Design review of the part built by this model. Coordinates are the model's own, in mm. Face numbers are marked on the shaded views. Coordinates: 2 decimals unless noted, no trailing zeros. Write each loop counter-clockwise with the first axis right and the second up, starting at its lowest first coordinate (ties: lowest second). Pieces come first, ordered by that corner, then holes.
Q1. The part is to be moulded in two halves that separate along X. For the marked faces 1, 2 and 3, say which applies: +X half, -X half, draft (parallel to the pull), parting line (faces both ways), or undercut.
Q2. Clearance check with flat-ended pins moving along their axes: pin 1 Ø1.6 at (x, z) = (-43, 35) entering from +Y; pin 2 Ø1.5 at (x, y) = (-95, 1) entering from -Z; pin 3 Ø1 at (y, z) = (-0.5, 27) entering from +X; pin 4 Ø1.5 at (x, y) = (-46, -1.5) entering from -Z. State where each tip first meets the part, or that it passes through.
Q3. Add section D-D, the plane x = -70. Give the boundary of the cut face in (y, z), plus the area to 3 significant figures.
Q4. To check wall thickness, follow probe 1 along Z at (x, y) = (-43, 0.65); probe 2 along X at (y, z) = (0.85, 35); probe 3 along Z at (x, y) = (-89.5, -1.6). State the ranges of each line that lie inside material, in increasing order.
Q5. Add section B-B, the plane y = -0.3. Give the boundary of the cut face in (x, z), plus the area to 3 significant figures.
Q6. Add section C-C, the plane z = 7. Give the boundary of the cut face in (x, y), plus the area to 3 significant figures.
Q7. Add section A-A, the plane x = -103. Give the boundary of the cut face in (y, z).
from build123d import *

# Parameters (mm, degrees)
SKETCH_R     = 1
PAD_DEPTH    = 4
POCKET_DEPTH = 0.5


with BuildPart() as part:
    # Sketch → Pad (new body)
    with BuildSketch(Plane(origin=(-43, 2, 10), x_dir=(-1, 0, 0), z_dir=(0, -1, 0))):
        with BuildLine():
            ThreePointArc((1.369567, -6.241771), (-2.39195, -6.793979), (-3.992648, -10.242416))
            Line((-3.992648, -10.242416), (-3.999699, -25.049081))
            ThreePointArc((-3.999699, -25.049081), (0.10526, -28.998615), (3.996742, -24.838581))
            Line((3.996742, -24.838581), (6.436421, -15.831628))
            ThreePointArc((10.468861, -13.107373), (8.040921, -13.860073), (6.436421, -15.831628))
            ThreePointArc((10.468861, -13.107373), (37.233561, -5.679802), (61.911635, 7.068166))
            ThreePointArc((61.911635, 7.068166), (63.070989, 11.678996), (58.563715, 13.191721))
            ThreePointArc((1.369567, -6.241771), (31.05105, 0.283484), (58.563715, 13.191721))
        make_face()
        with Locations((0, -10)):
            Circle(SKETCH_R, mode=Mode.SUBTRACT)
        with Locations((60, 10)):
            Circle(SKETCH_R, mode=Mode.SUBTRACT)
        with Locations((0, -25)):
            Circle(SKETCH_R, mode=Mode.SUBTRACT)
    extrude(amount=PAD_DEPTH)

    # Sketch001 → Pocket (cut)
    with BuildSketch(Plane(origin=(-43, -2, 10), x_dir=(-1, 0, 0), z_dir=(0, -1, 0))):
        with BuildLine():
            ThreePointArc((-0.032814, -13.479149), (2.709829, -12.250672), (3.417072, -9.329876))
            ThreePointArc((4.97037, -6.903931), (3.291608, -7.539293), (3.417072, -9.329876))
            ThreePointArc((4.97037, -6.903931), (30.091825, -0.923478), (53.929252, 9.007808))
            ThreePointArc((56.670903, 5.328015), (57.272793, 8.637695), (53.929252, 9.007808))
            ThreePointArc((9.344748, -11.398275), (33.841325, -5.393473), (56.670903, 5.328015))
            ThreePointArc((9.344748, -11.398275), (6.419172, -12.709963), (4.685346, -15.40688))
            Line((4.685346, -15.40688), (3.764189, -20.315398))
            ThreePointArc((-2.402749, -19.605513), (0.465776, -21.827722), (3.764189, -20.315398))
            Line((-2.489869, -16.419374), (-2.402749, -19.605513))
            ThreePointArc((-0.032814, -13.479149), (-1.889204, -14.424576), (-2.489869, -16.419374))
        make_face()
    extrude(amount=-POCKET_DEPTH, mode=Mode.SUBTRACT)


solid = part.part
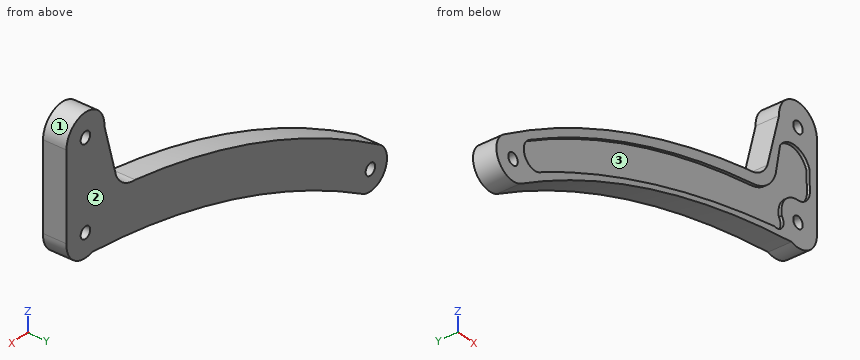
Here are the results:
1. face 1: parting line
1. face 2: draft
1. face 3: undercut
2. pin 1: passes through
2. pin 2: stops at z = 0.18
2. pin 3: stops at x = -39
2. pin 4: stops at z = 15.97
3. outline: (-2, 11.02) - (2, 11.02) - (2, 19.23) - (-2, 19.23) - (-2, 17.6) - (-1.5, 17.6) - (-1.5, 11.89) - (-2, 11.89) - close
3. area: 30.0 mm2
4. probe 1: z = 16 to 19, 21 to 34, 36 to 39
4. probe 2: x = -47 to -44, -42 to -39
4. probe 3: z = 3.39 to 4.58, 10.14 to 11.64
5. outline: (-104.91, 2.93) arc R3.5 ccw to (-101.56, -3.19) arc R137 cw to (-44.37, 16.24) arc R4 ccw to (-39.01, 20.24) - (-39, 35.05) arc R4 ccw (long way) to (-47, 34.84) - (-49.44, 25.83) arc R4.39 cw to (-53.47, 23.11) arc R135 ccw to start; hole circle Ø2 at (-103, 0); hole circle Ø2 at (-43, 20); hole circle Ø2 at (-43, 35)
5. area: 660 mm2
6. outline: (-98.29, -2) - (-95.6, -2) - (-95.6, -1.5) - (-83.84, -1.5) - (-83.84, -2) - (-81.36, -2) - (-81.36, 2) - (-98.29, 2) - close
6. area: 61.9 mm2
7. outline: (-2, -3.5) - (2, -3.5) - (2, -1) - (-2, -1) - close; (-2, 1) - (2, 1) - (2, 4.16) - (-2, 4.16) - close
